```python
from build123d import *

# Parameters (mm, degrees)
EXTRUDE1_DEPTH = 15
HOLE1_D        = 5
HOLE1_DEPTH    = 15
HOLE1_TIP      = 1.502151548


with BuildPart() as part:
    # Sketch1 → Extrude1 (new body)
    with BuildSketch(Plane.XY):
        with BuildLine():
            Line((-6.785898385, 0), (6.785898385, 0))
            ThreePointArc((6.785898385, 0), (7.785898385, -0.267949192), (8.517949192, -1))
            ThreePointArc((8.517949192, -1), (10.76763809, -1.931851653), (12.25, 0))
            Line((12.25, 0), (12.25, 32))
            ThreePointArc((12.25, 32), (13.128679656, 34.121320344), (15.25, 35))
            Line((15.25, 35), (31.179555311, 35))
            ThreePointArc((31.179555311, 35), (32.735875086, 34.564735612), (33.840587811, 33.38524584))
            Line((33.840587811, 33.38524584), (41.748237339, 18.19479243))
            ThreePointArc((41.748237339, 18.19479243), (42.075788934, 17.071013818), (41.948355691, 15.907429191))
            Line((41.948355691, 15.907429191), (40.144120894, 10.185127487))
            ThreePointArc((40.144120894, 10.185127487), (40.016687652, 9.02154286), (40.344239247, 7.897764249))
            Line((40.344239247, 7.897764249), (86.160656367, -80.11475416))
            ThreePointArc((86.160656367, -80.11475416), (86.064359479, -83.056319774), (83.499623867, -84.5))
            Line((83.499623867, -84.5), (16.854681642, -84.5))
            ThreePointArc((16.854681642, -84.5), (15.242782817, -84.030174337), (14.135758281, -82.767854785))
            Line((14.135758281, -82.767854785), (-5.282057281, -41.126214931))
            ThreePointArc((-5.282057281, -41.126214931), (-5.974210019, -40.182237706), (-6.974920212, -39.574991854))
            Line((-6.974920212, -39.574991854), (-12.931340914, -37.407032016))
            ThreePointArc((-12.931340914, -37.407032016), (-13.701027508, -36.991138005), (-14.317998731, -36.370870489))
            Line((-14.317998731, -36.370870489), (-30.648379548, -14.271904325))
            ThreePointArc((-30.648379548, -14.271904325), (-35.74299388, -4.421252914), (-37.5, 6.52878626))
            Line((-37.5, 6.52878626), (-37.5, 32))
            ThreePointArc((-37.5, 32), (-36.621320344, 34.121320344), (-34.5, 35))
            Line((-34.5, 35), (-15.25, 35))
            ThreePointArc((-15.25, 35), (-13.128679656, 34.121320344), (-12.25, 32))
            Line((-12.25, 32), (-12.25, 0))
            ThreePointArc((-12.25, 0), (-10.76763809, -1.931851653), (-8.517949192, -1))
            ThreePointArc((-8.517949192, -1), (-7.785898385, -0.267949192), (-6.785898385, 0))
        make_face()
    extrude(amount=EXTRUDE1_DEPTH)

    # Hole1
    with Locations(Plane(origin=(0, 35, 0), x_dir=(-1, 0, 0), z_dir=(0, 1, 0))):
        with Locations((-22, 7.5), (22, 7.5)):
            Hole(HOLE1_D / 2, depth=HOLE1_DEPTH)
            with Locations((0, 0, -(HOLE1_DEPTH + HOLE1_TIP / 2))):  # 118° drill point
                Cone(0, HOLE1_D / 2, HOLE1_TIP, mode=Mode.SUBTRACT)


solid = part.part
```
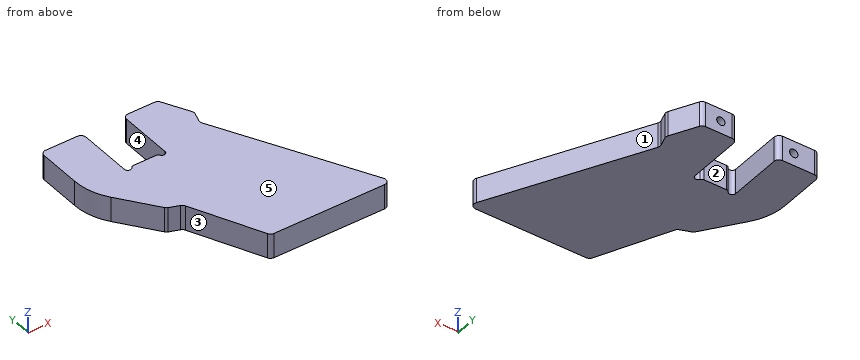
Model file for the job. Use its own axes, mm. Face numbers are marked on the shaded views. A direction names the side the tool comes from. Coordinates: 2 decimals unless noted, no trailing zeros. Loops run counter-clockwise (first coordinate to the right, second up) from the corner with the lowest first, then second, coordinate; pieces in that order, holes last. Notation, with made-up numbers: (-36.5, -37.75) - (-21.5, -37.75) arc R27 ccw to (-21.5, -3.75) - close; hole circle Ø7 at (5.5, -28). An arc over 180 degrees is marked (long way). Answer as a JSON object with one key per item and string values. Group by question number.
(1) Two-plate mould, pull along X, no slides. Class the marked faces 1, 2 and 3: released by +X, released by -X, zero draft, split by the parting line, or undercut.
(2) Tool access for the marked faces 4 and 5: list every direction of +Z, -Z, +X, -X, +Y, -Y with a clear straight run to the whole face (end or side of a thin tool).
(3) Probe line 1 along Z through (x, y) = (-22, 23.5); line 2 along X through (y, z) = (28.5, 7.5); line 3 along X through (y, z) = (30.25, 7.5). List the from-to ranges inside material, lowest first.
(4) Cut at A-A (x = 53). Give the cut face in (y, z).
(5) Flat gauge pins, fed straight in: pin 1 (4 mm diameter, centred on y = -51, z = 3, fed in from -X); pin 2 (7.5 mm diameter, centred on y = 23, z = 10, fed in from +X); pin 3 (2 mm diameter, centred on y = -48.5, z = 3.5, fed in from +X). Where does each tip first touch, or does it go through?
(6) Cut at B-B (y = -47). Give the cut face in (x, z).
Geometry says:
{
 "1": {"face 1": "released by +X", "face 2": "undercut", "face 3": "released by -X"},
 "2": {"face 4": "+Z, -Z, +Y", "face 5": "+Z, +X, -X, +Y, -Y"},
 "3": {"line 1": "z = 0 to 5, 10 to 15", "line 2": "x = -37.5 to -24.5, -19.5 to -12.25, 12.25 to 19.5, 24.5 to 36.38", "line 3": "x = -37.5 to -24.5, -19.5 to -12.25, 12.25 to 19.5, 24.5 to 35.47"},
 "4": {"outline": "(-84.5, 0) - (-16.41, 0) - (-16.41, 15) - (-84.5, 15) - close"},
 "5": {"pin 1": "stops at x = -1.61", "pin 2": "stops at x = 41.2", "pin 3": "stops at x = 70.22"},
 "6": {"outline": "(-2.54, 0) - (68.92, 0) - (68.92, 15) - (-2.54, 15) - close"}
}
